```python
from build123d import *


with BuildPart() as part:
    # Sketch1 → Revolve1 (revolve)
    with BuildSketch(Plane(origin=(0, 0, 0), x_dir=(0, 0, -1), z_dir=(1, 0, 0))):
        with BuildLine():
            Line((0, 0), (0, -22))
            Line((0, -22), (11, -22))
            Line((11, -22), (11, 0))
            Line((11, 0), (12.5, 0))
            Line((12.5, 0), (12.5, 3))
            Line((12.5, 3), (8, 3))
            Line((8, 3), (8, 6))
            Line((8, 6), (15, 6))
            Line((15, 6), (15, 9))
            ThreePointArc((15, 9), (7.762087348, 11.982827555), (0, 13))
            Line((0, 13), (0, 0))
        make_face()
    revolve(axis=Axis((0, 0, 0), (0, 1, 0)))


solid = part.part
```
Model file for the job. Use its own axes, mm. A direction names the side the tool comes from. Round coordinates to 2 decimals unless told otherwise and drop trailing zeros. Loops run counter-clockwise (first coordinate to the right, second up) from the corner with the lowest first, then second, coordinate; pieces in that order, holes last. Notation, with made-up numbers: M -5.5,-27 L 3.5,-27 A12 cw 3.5,-12 Z; hole C 29,3.25 d11. An arc over 180 degrees is marked long. Put each result on its own line as item: value. Start each with the question number.
Item 1: Cut at C-C (x = 0). List the corners of the cut face in (y, z) (3 decimals), then the cut area to 3 significant figures.
Item 2: Drill centre lines: line 1 along Y through (x, z) = (2.75, 11); line 2 along X through (y, z) = (-15, -9); line 3 along X through (y, z) = (-0.5, -7.5). Where is each one in solid material? Low to high.
Item 3: Cut at B-B (z = 0). List the corners of the cut face in (x, y) (3 decimals).
Item 4: 3-axis set-ups, long thin cutter, end or side, ignore diameter. For faces 1 (the face through (0, -22, 0)), 2 (the face through (6, 6, 6)), 3 (the face through (-3.755, 1.521, -11.923)): which of +Z, -Z, +X, -X, +Y, -Y reach the whole face in a straight line?
Item 5: Cut at A-A (x = -10). List the corners of the cut face in (y, z) (3 decimals).
Item 6: Cut at D-D (z = 8.5). List the corners of the cut face in (x, y) (3 decimals).
Item 7: Drop flat-ended pins along their axis: P1, Ø8, axis at x = 8.5, z = 8, coming from the +Y side; P2, Ø12, axis at y = -11, z = -5.5, coming from the -X side; P3, Ø5, axis at y = -12.5, z = -10.5, coming from the -X side. Give the stop position or say it passes through.
Answer block:
1. outline: M -22,-11 L 0,-11 L 0,-12.5 L 3,-12.5 L 3,-8 L 6,-8 L 6,-15 L 9,-15 A30.125 ccw 9,15 L 6,15 L 6,8 L 3,8 L 3,12.5 L 0,12.5 L 0,11 L -22,11 Z
1. area: 778 mm2
2. line 1: 0 to 3, 6 to 10.78
2. line 2: -6.32 to 6.32
2. line 3: -8.05 to 8.05
3. outline: M -15,6 L -8,6 L -8,3 L -12.5,3 L -12.5,0 L -11,0 L -11,-22 L 11,-22 L 11,0 L 12.5,0 L 12.5,3 L 8,3 L 8,6 L 15,6 L 15,9 A30.125 ccw -15,9 Z
4. face 1: +Z, -Z, +X, -X, -Y
4. face 2: none
4. face 3: -Y
5. outline: M -22,-4.583 L 0,-4.583 L 0,-7.5 L 3,-7.5 L 3,7.5 L 0,7.5 L 0,4.583 L -22,4.583 Z; M 6,-11.18 L 9,-11.18 A28.417 ccw 9,11.18 L 6,11.18 Z
6. outline: M -12.359,6 L 12.359,6 L 12.359,9 A28.901 ccw -12.359,9 Z; M -9.165,0 L -6.982,0 L -6.982,-22 L 6.982,-22 L 6.982,0 L 9.165,0 L 9.165,3 L -9.165,3 Z
7. P1: y = 12.01
7. P2: x = -11
7. P3: x = -7.55
